Can you work these out from the model? Positions are in its coordinate system, mm. Face numbers are marked on the shaded views. Give positions to 0.01 mm unless a question says otherwise; leave off trailing zeros. Loops run counter-clockwise (first coordinate to the right, second up) from the corner with the lowest first, then second, coordinate; pieces in that order, holes last. Notation, with made-up numbers: (11, 56.25) - (56, 56.25) arc R26 ccw to (56, 86.25) - close; hole circle Ø2 at (14, 83). An arc over 180 degrees is marked (long way). Write item = value, one per line.
Autodesk Fusion 360 part; units mm, degrees
sketch "Sketch1" plane through (0, 0, 0) normal (0, 0, 1) x (1, 0, 0)
  line L0 (0, 0) -> (100, 0)
  line L1 (100, 0) -> (100, 10)
  line L2 (100, 10) -> (0, 10)
  line L3 (0, 10) -> (0, 0)
  dimension "d1" = 100
  dimension "d2" = 10
extrude "Extrude1" add sketch "Sketch1" along normal blind 10
sketch "Sketch2" plane through (0, 0, 10) normal (0, 0, 1) x (-1, 0, 0)
  line L0 (0, -10) -> (0, 0)
  line L1 (0, 0) -> (-100, 0)
  line L2 (-100, 0) -> (-100, -10)
  line L3 (-100, -10) -> (0, -10)
  circle A0 centre (-5, -5) radius 4.5
  circle A1 centre (-25, -5) radius 4.5
  circle A2 centre (-45, -5) radius 4.5
  circle A3 centre (-65, -5) radius 4.5
  circle A4 centre (-85, -5) radius 4.5
  dimension "d5" = 9
  dimension "d6" = 9
  dimension "d7" = 9
  dimension "d8" = 9
  dimension "d9" = 9
extrude "Extrude2" cut sketch "Sketch2" against normal blind 20 contours A0 | A1 | A2 | A3 | A4
sketch "Sketch3" plane through (0, 0, 0) normal (0, -1, 0) x (1, 0, 0)
  line L0 (0, 0) -> (100, 0)
  line L1 (100, 0) -> (100, 10)
  line L2 (100, 10) -> (0, 10)
  line L3 (0, 10) -> (0, 0)
  circle A0 centre (75, 5) radius 4.5
  circle A1 centre (55, 5) radius 4.5
  circle A2 centre (35, 5) radius 4.5
  circle A3 centre (15, 5) radius 4.5
  dimension "d12" = 9
  dimension "d13" = 9
  dimension "d14" = 9
  dimension "d15" = 9
extrude "Extrude3" cut sketch "Sketch3" against normal blind 10 contours A0 | A1 | A2 | A3
sketch "Sketch4" plane through (100, 0, 0) normal (1, 0, 0) x (0, 1, 0)
  line L0 (0, 0) -> (10, 0)
  line L1 (10, 0) -> (10, 10)
  line L2 (10, 10) -> (0, 10)
  line L3 (0, 10) -> (0, 0)
  circle A0 centre (5, 5) radius 4
  dimension "d18" = 8
extrude "Extrude4" cut sketch "Sketch4" against normal blind 3 contours A0
sketch "Sketch5" plane through (0, 0, 0) normal (1, 0, 0) x (0, 1, 0)
  circle A0 centre (5, 5) radius 4
  circle A1 centre (5, 5) radius 3.5
  dimension "d21" = 8
  dimension "d22" = 7
extrude "Extrude5" add sketch "Sketch5" against normal blind 3
extrude "Extrude6" add 1 faces at (-3, 8.8054, 4.6274) along direction (1, 0, 0) blind 3
extrude "Extrude7" add 1 faces at (-3, 8.8054, 4.6274) along direction (1, 0, 0) blind 3
extrude "Extrude8" cut 1 faces at (-3, 8.8054, 4.6274) along direction (1, 0, 0) blind 3.5
extrude "Extrude9" add 2 faces at (0.5, 5.3558, 8.8079) (0.5, 5.3558, 8.8079) along direction (-1, 0, 0) blind 0.5
sketch "Sketch6" plane through (0, 0, 0) normal (-1, 0, 0) x (0, -1, 0)
  line L0 (-10, 0) -> (0, 0)
  line L1 (0, 0) -> (0, 10)
  line L2 (0, 10) -> (-10, 10)
  line L3 (-10, 10) -> (-10, 0)
  circle A0 centre (-5, 5) radius 4.5
  circle A1 centre (-5, 5) radius 4
  dimension "d33" = 9
  dimension "d34" = 8
sketch "Sketch7" plane through (0, 0, 0) normal (-1, 0, 0) x (0, -1, 0)
extrude "Extrude10" add sketch "Sketch6" along normal blind 3 contours A0
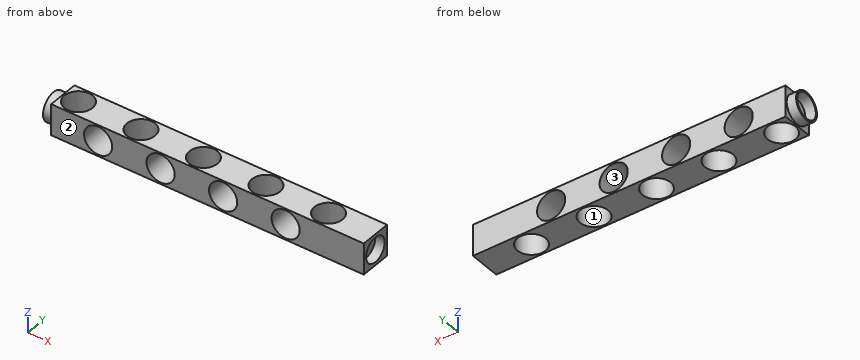
Q1. We'd pull the mould along X, two halves only. Please class the marked faces 1, 2 and 3: released by +X, released by -X, zero draft, split by the parting line, or undercut.
Output:
face_1 = undercut
face_2 = zero draft
face_3 = undercut
Q2. For pin 1 (3 mm diameter, centred on y = 5.5, z = 4, fed in from -X), with a flat end and sliding along its axis, tell me the tip position at first contact or that it passes through.
Output:
pin_1 = 0
Q3. I need wall thicknesses on L1, parallel to Y at x = 65, z = 4.75; L2, parallel to Z at x = -0.65, y = 5. Which ranges of each line are inside material? Lowest first, please.
Output:
L1 = 0 to 0.5, 9.5 to 10
L2 = 0.5 to 1, 9 to 9.5
Q4. Imagine slicing it at B-B, the plane x = 75. Write out the boundary of the cut face in (y, z).
Output:
outline = (0, 0) - (10, 0) - (10, 0.5) - (0, 0.5) - close; (0, 9.5) - (10, 9.5) - (10, 10) - (0, 10) - close
